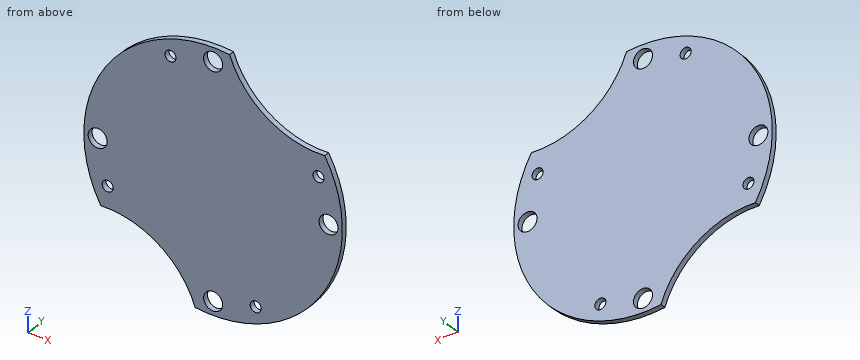
```python
from build123d import *

# Parameters (mm, degrees)
SKETCH1_R           = 37.5
BOSS_EXTRUDE1_DEPTH = 1.6
SKETCH3_R           = 1.6
SKETCH3_R_2         = 2.75
CUT_EXTRUDE1_DEPTH  = 10
SKETCH6_R           = 27.729942467
CUT_EXTRUDE2_DEPTH  = 10


with BuildPart() as part:
    # Sketch1 → Boss-Extrude1 (new body)
    with BuildSketch(Plane(origin=(0, 0, 0), x_dir=(1, 0, 0), z_dir=(0, 1, 0))):
        with Locations(Location((9.035122573, 0.49610085, 0), (0, 0, 270))):
            Circle(SKETCH1_R)
    extrude(amount=BOSS_EXTRUDE1_DEPTH)

    # Sketch3 → Cut-Extrude1 (cut)
    with BuildSketch(Plane(origin=(0, 1.6, 0), x_dir=(1, 0, 0), z_dir=(0, 1, 0))):
        with Locations(Location((-3.32689501, -30.094686593, 0), (0, 0, 270))):
            Circle(SKETCH3_R)
        with Locations(Location((-24.459801803, 0.49610085, 0), (0, 0, 270))):
            Circle(SKETCH3_R_2)
        with Locations(Location((9.035122573, 33.991025226, 0), (0, 0, 270))):
            Circle(SKETCH3_R_2)
        with Locations(Location((42.530046949, 0.49610085, 0), (0, 0, 270))):
            Circle(SKETCH3_R_2)
        with Locations(Location((9.035122573, -32.998823526, 0), (0, 0, 270))):
            Circle(SKETCH3_R_2)
        with Locations(Location((-21.55566487, 12.858118433, 0), (0, 0, 270))):
            Circle(SKETCH3_R)
        with Locations(Location((21.397140156, 31.086888293, 0), (0, 0, 270))):
            Circle(SKETCH3_R)
        with Locations(Location((39.625910016, -11.865916733, 0), (0, 0, 270))):
            Circle(SKETCH3_R)
    extrude(amount=-CUT_EXTRUDE1_DEPTH, mode=Mode.SUBTRACT)

    # Sketch6 → Cut-Extrude2 (cut)
    with BuildSketch(Plane(origin=(0, 1.6, 0), x_dir=(1, 0, 0), z_dir=(0, 1, 0))):
        with Locations((39.912604148, -46.085156826)):
            Circle(SKETCH6_R)
        with Locations((-22.36020617, 46.729917134)):
            Circle(SKETCH6_R)
    extrude(amount=-CUT_EXTRUDE2_DEPTH, mode=Mode.SUBTRACT)


solid = part.part
```
Verification items for the finished model (mm, model axes). Give positions to 0.01 mm unless a question says otherwise; leave off trailing zeros. Loops run counter-clockwise (first coordinate to the right, second up) from the corner with the lowest first, then second, coordinate; pieces in that order, holes last. Notation, with made-up numbers: M 77,0 L 90,0 A28 ccw 90,37 Z; hole C 12,7 d2. An arc over 180 degrees is marked long. Return JSON: item names as keys, results as strings.
1) Section check D-D, the plane z = -22. Enter the section's corners in (x, y), and give its area (3 significant figures).
Findings:
{"outline": "M -9.82,0 L 39.76,0 L 39.76,1.6 L -9.82,1.6 Z", "area": "79.3 mm2"}
2) Section check A-A, the plane z = 0.5. Enter the section's corners in (x, y).
Findings:
{"outline": "M -28.45,0 L -27.02,0 L -27.02,1.6 L -28.45,1.6 Z; M -21.9,0 L 39.97,0 L 39.97,1.6 L -21.9,1.6 Z; M 45.09,0 L 46.52,0 L 46.52,1.6 L 45.09,1.6 Z"}
3) Gauge pin test, flat ends, axial feed: P1, Ø4, axis at x = -12.5, z = -12, coming from the -Y side; P2, Ø1.9, axis at x = 21.4, z = -31.09, coming from the +Y side. Record the tip position at first contact, or that the pin passes through.
Findings:
{"P1": "stops at y = 0", "P2": "passes through"}
4) Section check B-B, the plane y = 0.25. Count the separate pieces of the cut face and the enclosed holes in it, and give its area (3 significant figures).
Findings:
{"separate pieces": "1", "enclosed holes": "8", "area": "3,870 mm2"}
5) Material ranges on L1, parallel to Z at x = -20.5, y = 0.5; L2, parallel to Z at x = -24.5, y = 0.7; L3, parallel to X at y = 1.5, z = 33.5, recorded low to high. Write a range as [from, to].
Findings:
{"L1": "z = [-19.06, -14.06], [-11.66, 22.61]", "L2": "z = [-17.28, -3.25], [2.25, 16.29]", "L3": "x = [-6.79, 6.33], [11.74, 15.2]"}
6) Section check C-C, the plane x = 31.5. Enter the section's corners in (y, z).
Findings:
{"outline": "M 0,-30.52 L 1.6,-30.52 L 1.6,19.66 L 0,19.66 Z"}
